Part model, mm, in its own coordinate system. Round coordinates to 2 decimals unless told otherwise and drop trailing zeros. Write each loop counter-clockwise with the first axis right and the second up, starting at its lowest first coordinate (ties: lowest second). Pieces come first, ordered by that corner, then holes. Notation, with made-up numbers: (37.25, 17.5) -> (63.25, 17.5) arc R23 cw to (63.25, 49.5) -> close; hole circle Ø2 at (59, 32). An arc over 180 degrees is marked (long way). Use CSV: the item, a comma, the result in double quotes. Start each with the question number.
```python
from build123d import *

# Parameters (mm, degrees)
F1_DEPTH = 6.35
F3_DEPTH = 6.351


with BuildPart() as f1:
    # F0 (on Top) → F1 (new body)
    with BuildSketch(Plane.XY):
        with BuildLine():
            Line((64.0479785321, 45.3746123328), (63.8854764337, 45.3746123328))
            Line((63.8854764337, 45.3746123328), (2.2767815665, 0))
            Line((2.2767815665, 0), (-39.7214530308, -30.9315692797))
            ThreePointArc((-39.7214530308, -30.9315692797), (-39.8444384128, -31.0225247493), (-39.9677839364, -31.1129912262))
            ThreePointArc((-39.9677839364, -31.1129912262), (-80.1407322996, -34.3509043357), (-101.2207046151, 0))
            Line((-101.2207046151, 0), (-101.2207046151, 9.9341273308))
            ThreePointArc((-101.2207046151, 9.9341273308), (-106.7247502506, 15.4381729662), (-112.228795886, 9.9341273308))
            Line((-112.228795886, 9.9341273308), (-112.228795886, 0))
            ThreePointArc((-112.228795886, 0), (-97.0433078129, -35.6915315199), (-60.7969101261, -49.5003375864))
            Line((-60.7969101261, -49.5003375864), (-52.0564235031, -48.3813164917))
            ThreePointArc((-52.0564235031, -48.3813164917), (-42.7531679645, -45.3464600069), (-34.228034924, -40.5419804156))
            Line((-34.228034924, -40.5419804156), (-34.2284778363, -40.5419804156))
            Line((-34.2284778363, -40.5419804156), (-34.2273214057, -40.5414794451))
            Line((-34.2273214057, -40.5414794451), (-19.8154687348, -34.2982047457))
            ThreePointArc((-19.8154687348, -34.2982047457), (-16.7847778238, -32.1655358704), (-13.1560671025, -31.4133241773))
            ThreePointArc((-13.1560671025, -31.4133241773), (-11.5145721435, -31.5621218969), (-9.9265901442, -32.0036642296))
            Line((-9.9265901442, -32.0036642296), (30.5177745747, -48.6430156736))
            Line((30.5177745747, -48.6430156736), (74.522745552, -48.229868259))
            ThreePointArc((74.522745552, -48.229868259), (79.0697257066, -40.3110135201), (76.337517689, -31.5979010883))
            ThreePointArc((76.337517689, -31.5979010883), (75.6238074008, -30.083288758), (74.6402267249, -28.7282972671))
            Line((74.6402267249, -28.7282972671), (65.5481898023, -18.39660376))
            ThreePointArc((65.5481898023, -18.39660376), (63.2520758801, 9.4447724115), (74.6402267249, 34.9540724138))
            Line((74.6402267249, 34.9540724138), (74.6402267249, 35.0096798031))
            ThreePointArc((74.6402267249, 35.0096798031), (74.8701460848, 35.255569914), (75.088660103, 35.5116489692))
            ThreePointArc((75.088660103, 35.5116489692), (74.2807317817, 45.7182435688), (64.0479785321, 45.3746123328))
        make_face()
    extrude(amount=F1_DEPTH)

    # F2 (on face) → F3 (cut, through all)
    with BuildSketch(Plane.XY.offset(6.35)):
        Polygon((12.0820117015, 7.2215215266), (32.3011358824, -20.6074602199), (37.9280887206, -16.5192021861), (18.2175485278, 11.7403253342), align=None)
    extrude(amount=-F3_DEPTH, mode=Mode.SUBTRACT)


solid = f1.part
```
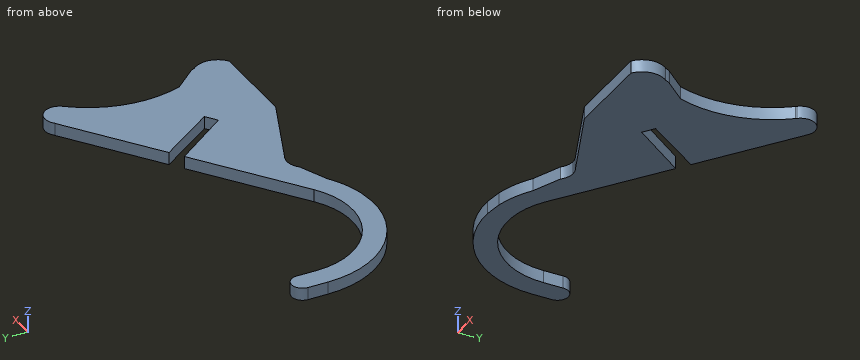
1. Flat gauge pins, fed straight in: pin 1 (1.5 mm diameter, centred on y = 11.5, z = 1, fed in from -X); pin 2 (1.5 mm diameter, centred on x = -31.5, z = 1, fed in from -Y); pin 3 (3 mm diameter, centred on x = -24, z = 1.5, fed in from -Y). Where does each tip first touch, or does it go through?
2. Band-saw the part on C-C (y = -23). List the corners of the cut face in (x, z).
3. Band-saw the part on D-D (x = -79). List the corners of the cut face in (y, z), then the cut area to 3 significant figures.
4. Band-saw the part on B-B (x = 28.5). List the corners of the cut face in (y, z).
5. Drill centre lines: line 1 along X through (y, z) = (-5.5, 1.25); line 2 along X through (y, z) = (1, 2); line 3 along Y through (x, z) = (36.5, 3). Where is each one in solid material? Low to high. Write a range as [from, to].
Answers below:
1,pin 1,"stops at x = -112.17"
1,pin 2,"stops at y = -39.68"
1,pin 3,"stops at y = -36.76"
2,outline,"(-106.57, 0) -> (-93.6, 0) -> (-93.6, 6.35) -> (-106.57, 6.35) -> close; (-28.95, 0) -> (69.6, 0) -> (69.6, 6.35) -> (-28.95, 6.35) -> close"
3,outline,"(-46.78, 0) -> (-34.91, 0) -> (-34.91, 6.35) -> (-46.78, 6.35) -> close"
3,area,"75.4 mm^2"
4,outline,"(-47.81, 0) -> (-15.38, 0) -> (-15.38, 6.35) -> (-47.81, 6.35) -> close; (-3, 0) -> (19.31, 0) -> (19.31, 6.35) -> (-3, 6.35) -> close"
5,line 1,"x = [-111.92, -100.83], [-5.19, 21.32], [30.24, 62.72]"
5,line 2,"x = [-112.23, -101.22], [3.63, 16.6], [25.71, 62.46]"
5,line 3,"y = [-48.59, -17.56], [-14.47, 25.21]"
